from build123d import *

# Parameters (mm, degrees)
CUT_EXTRUDE14_DEPTH = 0.561594
CIRPATTERN1_COUNT   = 6


with BuildPart() as part:
    # Sketch3 → Revolve1 (revolve)
    with BuildSketch(Plane(origin=(0, 0, 0), x_dir=(0, 0, -1), z_dir=(1, 0, 0)), mode=Mode.PRIVATE) as revolve1_sk:
        with BuildLine():
            Line((-3.68638517, 1.4224), (-3.68638517, 0.85344))
            ThreePointArc((-3.68638517, 0.85344), (-4.199806429, 0.946281688), (-4.6482, 1.21304783))
            Line((-4.6482, 1.21304783), (-6.35, 2.6924))
            Line((-6.35, 2.6924), (-6.35, 0))
            Line((-6.35, 0), (6.35, 0))
            Line((6.35, 0), (6.35, 1.4224))
            Line((6.35, 1.4224), (-3.68638517, 1.4224))
        make_face()
    revolve(revolve1_sk.sketch.rotate(Axis((0, 0, 6.35), (0, 0, -1)), 180), axis=Axis((0, 0, 6.35), (0, 0, -1)))

    # Sketch21 → Cut-Extrude14 (cut)
    with BuildSketch(Plane.XY.offset(6.35)):
        with BuildLine():
            Line((0, 0), (-0.53848, 0.932674719))
            ThreePointArc((-0.53848, 0.932674719), (-0.476327228, 0.965896068), (-0.412134749, 0.994981301))
            ThreePointArc((-0.412134749, 0.994981301), (0, 0.719601666), (0.412134749, 0.994981301))
            ThreePointArc((0.412134749, 0.994981301), (0.476327228, 0.965896068), (0.53848, 0.932674719))
            Line((0.53848, 0.932674719), (0, 0))
        make_face()
    cut_extrude14 = extrude(amount=-CUT_EXTRUDE14_DEPTH, mode=Mode.SUBTRACT)

    # CirPattern1: Cut-Extrude14 ×6 about axis
    cirpattern1_axis = Axis((0, 0, 0), (0, 0, 1))
    for i in range(1, CIRPATTERN1_COUNT):
        add(cut_extrude14.rotate(cirpattern1_axis, i * 360 / CIRPATTERN1_COUNT), mode=Mode.SUBTRACT)

    # Cut-Extrude15 cone 1 section (through the dimple's axis) → Cut-Extrude15 (revolve, cut)
    with BuildSketch(Plane(origin=(0, 0, 6.35), x_dir=(0, -1, 0), z_dir=(1, 0, 0))):
        Polygon((0, 0), (1.07696, 0), (0, 0.391981383), align=None)
    revolve(axis=Axis((0, 0, 6.35), (0, 0, -1)), mode=Mode.SUBTRACT)


solid = part.part
Input: part model. Units: mm. Frame: model coordinates. A direction names the side the tool comes from. Give positions to 0.01 mm unless a question says otherwise; leave off trailing zeros. Write each loop counter-clockwise with the first axis right and the second up, starting at its lowest first coordinate (ties: lowest second). Pieces come first, ordered by that corner, then holes. Notation, with made-up numbers: M 22,67.25 L 52,67.25 A17 ccw 52,77.25 Z; hole C 74,-3.75 d4. An arc over 180 degrees is marked long. Write item = value, one per line. Start each with the question number.
1) Cut plane B-B on z = 3.5. Return the cut outline in (x, y), then the cut area to 3 significant figures.
2) First-contact query: pin 1 Ø2 at (x, z) = (-1, -2) entering from -Y; pin 2 Ø2 at (y, z) = (-1, -3) entering from -X. Flat tips, straight axial feed; report the tip coordinate or a pass-through.
3) Reachability of faces 1 (the flat face through (0, 0, 5.788)), 2 (the cylindrical face through (1.26, -0.66, -1.26)), 3 (the flat face through (1, -1, 6.35)) from +Z, -Z, +X, -X, +Y, -Y: full face, straight path, thin tool, end or side. Return the list, or none.
4) Material intervals for line 1 along Z through (x, y) = (-0.95, -0.75); line 2 along Z through (x, y) = (0.5, -0.35); line 3 along X through (y, z) = (0.1, 3), sorted ascending. Write a range as [from, to].
5) Cut plane A-A on x = 0. Return the cut outline in (y, z), then the cut area to 3 significant figures.
Solved:
q1.outline = C 0,0 d2.84
q1.area = 6.36 mm2
q2.pin_1 = -1.42
q2.pin_2 = -1.42
q3.face_1 = +Z
q3.face_2 = -Z
q3.face_3 = +Z, +X, -X, +Y, -Y
q4.line_1 = [-6.35, 3.69], [4.65, 6.35]
q4.line_2 = [-6.35, 5.79]
q4.line_3 = [-1.42, 1.42]
q5.outline = M -2.69,6.35 L -1.21,4.65 A1.47 cw -0.85,3.69 L -1.42,3.69 L -1.42,-6.35 L 1.42,-6.35 L 1.42,3.69 L 0.85,3.69 A1.47 cw 1.21,4.65 L 2.69,6.35 L 1.08,6.35 L 0.72,6.22 L 0.72,5.79 L -0.72,5.79 L -0.72,6.22 L -1.08,6.35 Z
q5.area = 36.2 mm2
